Autodesk Inventor part; units mm, degrees
ref_plane "YZ Plane" through (0, 0, 0) normal (1, 0, 0) x (0, 1, 0)
ref_plane "XZ Plane" through (0, 0, 0) normal (0, 1, 0) x (-1, 0, 0)
ref_plane "XY Plane" through (0, 0, 0) normal (0, 0, 1) x (1, 0, 0)
sketch "Sketch1" plane through (0, 0, 0) normal (1, 0, 0) x (0, 1, 0)
  line L0 (-2.5, 12.5) -> (-5, 12.5)
  line L1 (5, -6.2) -> (5, 6.2)
  line L2 (-5, 12.5) -> (-5, 6.2)
  line L3 (-5, -6.2) -> (-5, -12.5)
  line L4 (-5, 6.2) -> (5, 6.2)
  line L5 (-5, -6.2) -> (5, -6.2)
  line L6 (7, -6.2) -> (7, 8.2)
  line L7 (5, 6.2) -> (5, -6.2)
  line L8 (5, 6.2) -> (-5, 6.2)
  line L9 (-5, 6.2) -> (-5, 8.2)
  line L10 (-2.5, 8.2) -> (7, 8.2)
  line L11 (7, 8.2) -> (7, 6.2)
  line L12 (-5, 6.2) -> (-2.5, 6.2)
  line L13 (-2.5, 8.2) -> (-2.5, 12.5)
  line L14 (-2.5, 12.5) -> (-5, 12.5)
  line L15 (-5, 12.5) -> (-5, 6.2)
  line L16 (5, 6.2) -> (5, 0)
  line L17 (5, 0) -> (-5.8889, 0)
  line L18 (-2.5, -12.5) -> (-5, -12.5)
  line L19 (5, 6.2) -> (5, -6.2)
  line L20 (-5, -12.5) -> (-5, -6.2)
  line L21 (-5, -6.2) -> (5, -6.2)
  line L22 (7, 6.2) -> (7, -8.2)
  line L23 (5, -6.2) -> (5, 6.2)
  line L24 (5, -6.2) -> (-5, -6.2)
  line L25 (-5, -6.2) -> (-5, -8.2)
  line L26 (-2.5, -8.2) -> (7, -8.2)
  line L27 (7, -8.2) -> (7, -6.2)
  line L28 (-5, -6.2) -> (-2.5, -6.2)
  line L29 (-2.5, -8.2) -> (-2.5, -12.5)
  line L30 (-2.5, -12.5) -> (-5, -12.5)
  line L31 (-5, -12.5) -> (-5, -6.2)
  line L32 (5, -6.2) -> (5, 0)
  dimension "d1" = 25
  dimension "d2" = 6.3
  dimension "d5" = 10
  dimension "d6" = 10
  dimension "d9" = 2
  dimension "d10" = 2.5
  dimension "d11" = 6.2
extrude "Extrusion1" add sketch "Sketch1" along normal blind 11
sketch "Sketch2" plane through (0, -2.5, 12.5) normal (0, 1, 0) x (1, 0, 0)
  line L0 (0, 4.3) -> (0, 0)
  line L1 (0, 0) -> (11, 0)
  line L2 (6.6, 0) -> (6.6, 3.5)
  line L3 (6.6, 3.5) -> (0, 3.5)
  point P0 (0, 12.5)
  dimension "d15" = 3.5
  dimension "d16" = 6.6
hole "Hole1" at (6.6, -2.5, 9) direction (0, -1, 0) diameter 1.7 depth 5.692
sketch "Sketch3" plane through (0, -2.5, -8.2) normal (0, 1, 0) x (1, 0, 0)
  line L0 (0, 4.3) -> (11, 4.3)
  line L1 (0, 4.3) -> (6.6, 4.3)
  line L2 (6.6, 4.3) -> (6.6, 0.8)
  line L3 (6.6, 4.3) -> (10.1, 4.3) construction
  point P0 (0, -8.2)
  dimension "d24" = 6.6
  dimension "d25" = 3.5
  dimension "d26" = 90
hole "Hole2" at (6.6, -2.5, -9) direction (0, -1, 0) diameter 1.7 depth 5.692
sketch "Sketch4" plane through (0, 7, 8.2) normal (0, 1, 0) x (1, 0, 0)
  arc A0 (6.3128, 0) -> (6.8872, 0) centre (6.6, -0.8) ccw
  arc A1 (6.8872, 16.4) -> (6.3128, 16.4) centre (6.6, 17.2) ccw
  point P0 (0, 8.2)
hole "Hole3" at (6.6, 7, 9) at (6.6, 7, -9) direction (0, -1, 0) diameter 4 depth 10
fillet "Fillet1" radius 1 6 edges at (2.3835, 7, -8.2) (2.3835, 7, 8.2) (9.7165, 7, 8.2) (9.7165, 7, -8.2) (5.5, -2.5, 12.5) (5.5, -2.5, -12.5)
sketch "Sketch5" plane through (0, 5, -6.2) normal (0, -1, 0) x (1, 0, 0)
  line L0 (11, 12.4) -> (11, 0)
  line L1 (0, 12.4) -> (11, 12.4)
  line L2 (11, 12.4) -> (10, 12.4)
  line L3 (10, 12.4) -> (6, 12.4)
  line L4 (0, 0) -> (11, 0)
  line L5 (10, 12.4) -> (6, 12.4)
  line L6 (6, 12.4) -> (6, 0)
  line L7 (6, 0) -> (10, 0)
  line L8 (10, 0) -> (10, 12.4)
  point P0 (0, 6.2)
  point P1 (10, 0)
  dimension "d42" = 1
  dimension "d43" = 4
extrude "Extrusion2" add sketch "Sketch5" along normal blind 0.5 contours L8 L4 L6 L1
fillet "Fillet2" radius 0.3 2 edges at (10, 4.5, 0) (6, 4.5, 0)
properties part number "soporte velo"
Can you work these out from the model? Positions are in its coordinate system, mm. A direction names the side the tool comes from. Coordinates: 2 decimals unless noted, no trailing zeros. Order: outer loops, then holes, each group sorted by start corner. A loop starts at its lowest first (then second) coordinate and runs counter-clockwise, first axis right, second up.
1. If we section it at A-A (x = 6.6): Please give me the cut outline in (y, z), then the cut area to 3 significant figures.
2. Thinking about a two-plate mould opening in Z: for faces 1 (the face through (5.577, -2.801, -12.215)), 2 (the face through (2, 2, 8.2)), 3 (the face through (6.926, -4.014, 9.785)), which applies, +Z half, -Z half, draft (parallel to the pull), parting line (faces both ways), or undercut?
3. If we section it at B-B (z = 9): Please give me the cut outline in (x, y).
4. For faces 4 (the face through (10, 2, -8.2)), 5 (the face through (5, -5, -9)), 6 (the face through (6.926, -4.014, -8.215)), 7 (the face through (6.512, 0.819, 7.002)), 8 (the face through (10, 2, 8.2)), which set-ups out of +Z, -Z, +X, -X, +Y, -Y let a thin tool reach every point of the face, with its end or its side?
5. I need wall thicknesses on line 1 (Z direction, x = 6.6, y = -3.7); line 2 (X direction, y = -3.55, z = -9); line 3 (Z direction, x = 6.6, y = 2). Which ranges of each line are inside material? Lowest first, please.
6. If we section it at C-C (y = -1.5): Please give me the cut outline in (x, z), then the cut area to 3 significant figures.
7. I'm going to push flat-ended pins straight in: pin 1 (4 mm diameter, centred on x = 2, y = 0.5, fed in from +Z); pin 2 (1 mm diameter, centred on x = 7.5, z = -0.5, fed in from -Y); pin 3 (1 mm diameter, centred on x = 7, z = 10.5, fed in from +Y). Where does each tip first touch, or does it pass through?
8. If we section it at D-D (x = 9.25): Please give me the cut outline in (y, z), then the cut area to 3 significant figures.
Entries:
1. outline: (-5, -12.5) - (-3.5, -12.5) arc R1 ccw to (-2.5, -11.5) - (-2.5, -11) - (-3, -11) - (-3, -9.85) - (-5, -9.85) - close; (-5, -8.15) - (-3, -8.15) - (-3, -7) - (7, -7) - (7, 7) - (-3, 7) - (-3, 8.15) - (-5, 8.15) - (-5, 6.2) - (4.5, 6.2) - (4.5, -6.2) - (-5, -6.2) - close; (-5, 9.85) - (-3, 9.85) - (-3, 11) - (-2.5, 11) - (-2.5, 11.5) arc R1 ccw to (-3.5, 12.5) - (-5, 12.5) - close
1. area: 66.5 mm2
2. face 1: -Z half
2. face 2: +Z half
2. face 3: undercut
3. outline: (0, -5) - (5.75, -5) - (5.75, -3) - (4.6, -3) - (4.6, -2.5) - (0, -2.5) - close; (7.45, -5) - (11, -5) - (11, -2.5) - (8.6, -2.5) - (8.6, -3) - (7.45, -3) - close
4. face 4: -Z, +X, -X, +Y
4. face 5: +Z, -Z, +X, -X, -Y
4. face 6: +Y, -Y
4. face 7: +Y
4. face 8: +Z, +X, -X, +Y
5. line 1: z = -12.5 to -9.85, -8.15 to -6.2, 6.2 to 8.15, 9.85 to 12.5
5. line 2: x = 0 to 5.75, 7.45 to 11
5. line 3: z = -7 to -6.2, 6.2 to 7
6. outline: (0, -8.2) - (4.77, -8.2) arc R2 cw to (8.43, -8.2) - (11, -8.2) - (11, -6.2) - (0, -6.2) - close; (0, 6.2) - (11, 6.2) - (11, 8.2) - (8.43, 8.2) arc R2 cw to (4.77, 8.2) - (0, 8.2) - close
6. area: 37.7 mm2
7. pin 1: stops at z = 8.2
7. pin 2: stops at y = 4.5
7. pin 3: stops at y = -2.5
8. outline: (-5, -12.5) - (-3.5, -12.5) arc R1 ccw to (-2.5, -11.5) - (-2.5, -8.2) - (6, -8.2) arc R1 ccw to (7, -7.2) - (7, 7.2) arc R1 ccw to (6, 8.2) - (-2.5, 8.2) - (-2.5, 11.5) arc R1 ccw to (-3.5, 12.5) - (-5, 12.5) - (-5, 6.2) - (4.5, 6.2) - (4.5, -6.2) - (-5, -6.2) - close
8. area: 99.6 mm2
